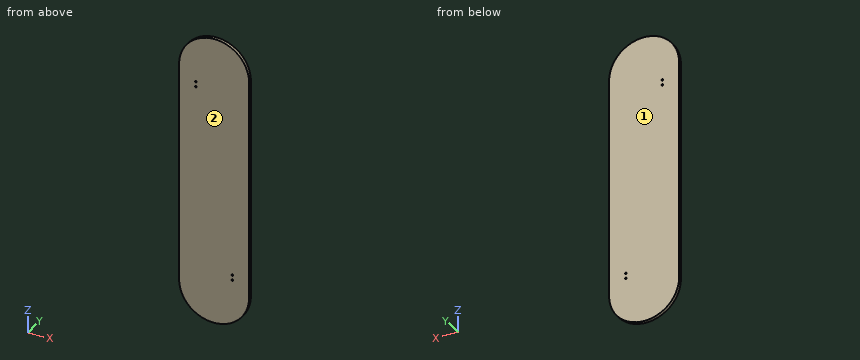
Autodesk Inventor part; units mm, degrees
ref_plane "YZ Plane" through (0, 0, 0) normal (1, 0, 0) x (0, 1, 0)
ref_plane "XZ Plane" through (0, 0, 0) normal (0, 1, 0) x (-1, 0, 0)
ref_plane "XY Plane" through (0, 0, 0) normal (0, 0, 1) x (1, 0, 0)
sketch "スケッチ1" plane through (0, 0, 0) normal (0, 1, 0) x (-1, 0, 0)
  point P0 (0, 0)
sketch "スケッチ2" plane through (0, 0, 0) normal (0, 1, 0) x (-1, 0, 0)
  line L0 (0.845, -60.969) -> (0.845, -330.969)
  line L1 (0, 0) -> (0, -1.5537)
  line L2 (-202.155, -60.969) -> (-202.155, -330.969)
  arc A0 (-202.155, -330.969) -> (0.845, -330.969) centre (-100.655, -330.969) ccw
  line L3 (0.845, -60.969) -> (0.845, 309.031)
  line L4 (-202.155, -60.969) -> (-202.155, 309.031)
  arc A1 (0.845, 309.031) -> (-202.155, 309.031) centre (-100.655, 309.031) ccw
  circle A2 centre (-47.655, 289.031) radius 6
  circle A3 centre (-47.655, 274.031) radius 6
  circle A4 centre (-153.655, -310.969) radius 6
  circle A5 centre (-153.655, -295.969) radius 6
  dimension "d0" = 270
  dimension "d1" = 203
  dimension "d38" = 12
  dimension "d39" = 20
  dimension "d40" = 12
  dimension "d41" = 15
  dimension "d42" = 48.5
  dimension "d43" = 48.5
  dimension "d44" = 12
  dimension "d45" = 12
  dimension "d46" = 20
  dimension "d47" = 15
  dimension "d48" = 48.5
  dimension "d49" = 48.5
extrude "押し出し1" add sketch "スケッチ2" against normal blind 10 contours L0 A0 L2 L4 A1 L3 | A2 | A3 | A4 | A5
sketch "スケッチ6" plane through (0, 0, 0) normal (0, 1, 0) x (1, 0, 0)
  circle A0 centre (153.655, 290.969) radius 6
  circle A1 centre (153.655, 275.969) radius 6
  arc A2 (202.155, 330.969) -> (-0.845, 330.969) centre (100.655, 330.969) ccw
  line L0 (202.155, 330.969) -> (202.155, -309.031)
  point P0 (0, 0)
  dimension "d50" = 12
  dimension "d51" = 12
  dimension "d52" = 40
  dimension "d53" = 48.5
  dimension "d54" = 48.5
  dimension "d55" = 15
hole "穴4" at (153.655, 0, -290.969) at (153.655, 0, -275.969) direction (0, -1, 0) diameter 4.917 end through all
sketch "スケッチ7" plane through (0, 0, 0) normal (0, 1, 0) x (1, 0, 0)
  circle A0 centre (47.655, -269.031) radius 6
  circle A1 centre (47.655, -254.031) radius 6
  line L0 (-0.845, -309.031) -> (-0.845, 330.969)
  arc A2 (-0.845, -309.031) -> (202.155, -309.031) centre (100.655, -309.031) ccw
  point P0 (0, 0)
  dimension "d63" = 12
  dimension "d64" = 12
  dimension "d65" = 48.5
  dimension "d66" = 48.5
  dimension "d67" = 40
  dimension "d68" = 15
hole "穴5" at (47.655, 0, 254.031) at (47.655, 0, 269.031) direction (0, -1, 0) diameter 4.917 end through all
properties part number "sfp_smartboard_upper_deck" material "合板、仕上げ"
Geometry check sheet. Reference: the model listing, model coordinates, mm. Face numbers are marked on the shaded views. Give positions to 0.01 mm unless a question says otherwise; leave off trailing zeros. Order: outer loops, then holes, each group sorted by start corner. A loop starts at its lowest first (then second) coordinate and runs counter-clockwise, first axis right, second up. Notation, with made-up numbers: (22.25, 15) - (74.25, 15) arc R18 ccw to (74.25, 25) - close; hole circle Ø7 at (-26, -17.75). An arc over 180 degrees is marked (long way). Write item = value, one per line. Start each with the question number.
1) Scan lines: L1, parallel to X at y = -0.75, z = -275.5 (3 decimals); L2, parallel to Z at x = 57.5, y = -0.25; L3, parallel to Z at x = 94.5, y = -2.75. Record each from-to range of solid material in increasing order.
2) Gauge pin test, flat ends, axial feed: pin 1 Ø4.5 at (x, z) = (47.655, 269.031) entering from +Y; pin 2 Ø2 at (x, y) = (119.5, -3.5) entering from -Z. Record the tip position at first contact, or that the pin passes through.
3) Section check B-B (z = 332). Enter the section's corners in (x, y).
4) Section check C-C (x = 172). Enter the section's corners in (y, z), then the cut area to 3 significant figures.
5) Draft check along Y on the marked faces 1 and 2. Enter one of: released by +Y, released by -Y, zero draft, split by the parting line, or undercut.
6) Section check A-A (y = -1.5). Enter the section's corners in (x, z) (1 decimal).
Geometry check:
q1.L1 = -0.845 to 151.242, 156.068 to 202.155
q1.L2 = -422.84 to 400.9
q1.L3 = -432.28 to 410.34
q2.pin_1 = through
q2.pin_2 = -430.89
q3.outline = (1.79, -10) - (199.52, -10) - (199.52, 0) - (1.79, 0) - close
q4.outline = (-10, -403.16) - (0, -403.16) - (0, 381.23) - (-10, 381.23) - close
q4.area = 7,840 mm2
q5.face_1 = released by +Y
q5.face_2 = released by -Y
q6.outline = (-0.8, -331) arc R101.5 ccw to (202.2, -331) - (202.2, 309) arc R101.5 ccw to (-0.8, 309) - close; hole circle Ø4.9 at (47.7, 254); hole circle Ø4.9 at (47.7, 269); hole circle Ø4.9 at (153.7, -291); hole circle Ø4.9 at (153.7, -276)
